```python
from build123d import *

# Parameters (mm, degrees)
BOSS_EXTRUDE1_DEPTH = 0.800000038
BOSS_EXTRUDE2_DEPTH = 1.200000057
CUT_EXTRUDE1_DEPTH  = 7.619101177


with BuildPart() as part:
    # Sketch1 → Boss-Extrude1 (new body)
    with BuildSketch(Plane.XY.offset(2.000000095)):
        Polygon((1.944495831, 2.910143696), (1.339392038, 3.233578522), (0.682816142, 3.432748606), (0, 3.500000108), (-0.682816142, 3.432748606), (-1.339392038, 3.233578522), (-1.944495831, 2.910143696), (-2.474873792, 2.474873792), (-2.910143696, 1.944495831), (-3.233578522, 1.339392038), (-3.432748606, 0.682816142), (-3.500000108, 0), (-3.432748606, -0.682816142), (-3.233578522, -1.339392038), (-2.910143696, -1.944495831), (-2.474873792, -2.474873792), (-1.944495831, -2.910143696), (-1.339392038, -3.233578522), (-0.682816142, -3.432748606), (0, -3.500000108), (0.682816142, -3.432748606), (1.339392038, -3.233578522), (1.944495831, -2.910143696), (2.474873792, -2.474873792), (2.910143696, -1.944495831), (3.233578522, -1.339392038), (3.432748606, -0.682816142), (3.500000108, 0), (3.432748606, 0.682816142), (3.233578522, 1.339392038), (2.910143696, 1.944495831), (2.474873792, 2.474873792), align=None)
    extrude(amount=-BOSS_EXTRUDE1_DEPTH)

    # Sketch2 → Boss-Extrude2 (add)
    with BuildSketch(Plane(origin=(0, 0, 1.200000057), x_dir=(-1, 0, 0), z_dir=(0, 0, -1))):
        Polygon((-5.249999929, -2.000000095), (-5.249999929, 2.000000095), (-2.864592476, 2.000000095), (-2.474873792, 2.474873792), (-1.944495831, 2.910143696), (-1.339392038, 3.233578522), (-0.682816142, 3.432748606), (0, 3.500000108), (0.682816142, 3.432748606), (1.339392038, 3.233578522), (1.944495831, 2.910143696), (2.474873792, 2.474873792), (2.910143696, 1.944495831), (3.233578522, 1.339392038), (3.432748606, 0.682816142), (3.500000108, 0), (3.432748606, -0.682816142), (3.233578522, -1.339392038), (2.910143696, -1.944495831), (2.474873792, -2.474873792), (1.944495831, -2.910143696), (1.339392038, -3.233578522), (0.682816142, -3.432748606), (0, -3.500000108), (-0.682816142, -3.432748606), (-1.339392038, -3.233578522), (-1.944495831, -2.910143696), (-2.474873792, -2.474873792), (-2.864592476, -2.000000095), align=None)
    extrude(amount=BOSS_EXTRUDE2_DEPTH)

    # Sketch3 → Cut-Extrude1 (cut, through all)
    with BuildSketch(Plane(origin=(0, 0, 0), x_dir=(-1, 0, 0), z_dir=(0, 0, -1))):
        Polygon((-1.472243224, 0.850000011), (-1.642073854, 0.439992378), (-1.700000023, 0), (-1.642073854, -0.439992378), (-1.472243224, -0.850000011), (-1.202081563, -1.202081563), (-0.850000011, -1.472243224), (-0.439992378, -1.642073854), (0, -1.700000023), (0.439992378, -1.642073854), (0.850000011, -1.472243224), (1.202081563, -1.202081563), (1.472243224, -0.850000011), (1.642073854, -0.439992378), (1.700000023, 0), (1.642073854, 0.439992378), (1.472243224, 0.850000011), (1.202081563, 1.202081563), (0.850000011, 1.472243224), (0.439992378, 1.642073854), (0, 1.700000023), (-0.439992378, 1.642073854), (-0.850000011, 1.472243224), (-1.202081563, 1.202081563), align=None)
    extrude(amount=-CUT_EXTRUDE1_DEPTH, mode=Mode.SUBTRACT)


solid = part.part
```
Geometry check sheet. Reference: the model listing, model coordinates, mm. A direction names the side the tool comes from. Round coordinates to 2 decimals unless told otherwise and drop trailing zeros. Order: outer loops, then holes, each group sorted by start corner. A loop starts at its lowest first (then second) coordinate and runs counter-clockwise, first axis right, second up. Notation, with made-up numbers: M -38.5,4.25 L -29.5,4.25 A31 ccw -29.5,33.25 Z; hole C 55,-13 d11. An arc over 180 degrees is marked long. Write item = value, one per line.
Q1. Section check B-B (x = 0.25). Enter the section's corners in (y, z).
Answer block:
outline = M -3.48,0 L -1.67,0 L -1.67,2 L -3.48,2 Z; M 1.67,0 L 3.48,0 L 3.48,2 L 1.67,2 Z
Q2. Section check C-C (x = 4.25). Enter the section's corners in (y, z).
Answer block:
outline = M -2,0 L 2,0 L 2,1.2 L -2,1.2 Z
Q3. Depth check by flat-ended pin: pin 1 Ø1 at (x, z) = (-1, 0) entering from -Y; pin 2 Ø1 at (x, z) = (4.5, 0.5) entering from +Y; pin 3 Ø1 at (x, z) = (4, 0.5) entering from -Y. Enter the tip coordinate at first touch or a pass-through.
Answer block:
pin_1 = -3.45
pin_2 = 2
pin_3 = -2
Q4. Section check A-A (y = -0.25). Enter the section's corners in (x, z), plus the area to 3 significant figures.
Answer block:
outline = M -3.48,0 L -1.67,0 L -1.67,2 L -3.48,2 Z; M 1.67,0 L 5.25,0 L 5.25,1.2 L 3.48,1.2 L 3.48,2 L 1.67,2 Z
area = 9.36 mm^2
Q5. Set-up check for faces 4 (the flat face through (4, -2, 1)), 5 (the flat face through (2, 1, 2)), 6 (the flat face through (4, 2, 1)): record each of +Z, -Z, +X, -X, +Y, -Y from which the full face is reachable in a straight line by a thin tool's end or side.
Answer block:
face_4 = +Z, -Z, +X, -Y
face_5 = +Z, +X, -X, +Y, -Y
face_6 = +Z, -Z, +X, +Y
Q6. Section check D-D (y = 1). Enter the section's corners in (x, z), plus the area to 3 significant figures.
Answer block:
outline = M -3.34,0 L -1.36,0 L -1.36,2 L -3.34,2 Z; M 1.36,0 L 5.25,0 L 5.25,1.2 L 3.34,1.2 L 3.34,2 L 1.36,2 Z
area = 10.2 mm^2
Q7. Scan lines: line 1 (X direction, y = 0.25, z = 1.65); line 2 (X direction, y = 1.25, z = 0.3). Record each from-to range of solid material in increasing order.
Answer block:
line_1 = -3.48 to -1.67, 1.67 to 3.48
line_2 = -3.26 to -1.14, 1.14 to 5.25
Q8. Release check for a two-part mould opening along Z. For faces 1 (the flat face through (5.25, 0, 1)), 2 (the flat face through (2, 0, 0)), 3 (the flat face through (4, 0, 1.2)) record: released by +Z, released by -Z, zero draft, split by the parting line, or undercut.
Answer block:
face_1 = zero draft
face_2 = released by -Z
face_3 = released by +Z
